The listing builds one solid part. Answer for the finished solid, in the listing's coordinates (mm). A direction names the side the tool comes from. Give positions to 0.01 mm unless a question says otherwise; leave off trailing zeros. Write each loop counter-clockwise with the first axis right and the second up, starting at its lowest first coordinate (ties: lowest second). Pieces come first, ordered by that corner, then holes. Notation, with made-up numbers: (41.25, -15) - (56.25, -15) arc R32 cw to (56.25, 14) - close; hole circle Ø10 at (24.25, 3.5). An arc over 180 degrees is marked (long way). Write each question's results on one line, items separated by ' | '. Start each with the question number.
Q1. Flat-ended cylindrical pins translate along their axes: pin 1 Ø2 at (x, z) = (-1.5, 4.5) entering from -Y; pin 2 Ø1.5 at (x, z) = (28, 3) entering from +Y. Find the tip coordinate at first contact, or state that the pin passes through.
Q2. Section C-C (z = 1.9) is taken. Determine the outline of the cut face in (x, y).
Q3. Find the intervals of material crossed by probe 1 along Y at (x, z) = (0, 2.65); probe 2 along X at (y, z) = (0.5, 0.45); probe 3 along Y at (x, z) = (-2.5, 2.2), in increasing order.
Q4. Section A-A (x = 0) is taken. Determine the outline of the cut face in (y, z).
Q5. Section B-B (y = 2) is taken. Determine the outline of the cut face in (x, z).
Q6. For a pull along Y with two mould halves and no side action, classify faces 4 (the face through (23.142, -22, 2)), 5 (the face through (27, 28.492, 2)), 6 (the face through (9.67, -18.593, 2.535)) as pulls with the +Y half, pulls with the -Y half, needs draft (parallel to the pull), parting line crosses it, or undercut.
Q7. For faces 1 (the face through (23.142, 23, 2)), 2 (the face through (27, -27.794, 2)), 3 (the face through (-19.24, 19.96, 2.54)), determine the directions among +Z, -Z, +X, -X, +Y, -Y from which every point of the face is accessible in a straight line to the end or side of a thin tool.
```python
from build123d import *

# Parameters (mm, degrees)
F0_R     = 28.827608
F1_DEPTH = 5
F2_R     = 20.957085
F3_DEPTH = 5
F4_W     = 7.907964
F4_H     = 56.286104
F5_DEPTH = 5
F6_R     = 2.590527
F7_DEPTH = 5


with BuildPart() as f1:
    # F0 (on Top) → F1 (new body)
    with BuildSketch(Plane.XY):
        with Locations((0, 0.851326)):
            Circle(F0_R)
    extrude(amount=F1_DEPTH)

    # F2 (on face) → F3 (cut)
    with BuildSketch(Plane.XY.offset(5)):
        Circle(F2_R)
    extrude(amount=-F3_DEPTH, mode=Mode.SUBTRACT)

    # F4 (on Top) → F5 (join)
    with BuildSketch(Plane.XY):
        with Locations((27.096411, 0.348881)):
            Rectangle(F4_W, F4_H)
    extrude(amount=F5_DEPTH)

    # F6 (on face) → F7 (cut)
    with BuildSketch(Plane.XY.offset(5)):
        with Locations((-16.652713, 19.845931)):
            Circle(F6_R)
    extrude(amount=-F7_DEPTH, mode=Mode.SUBTRACT)


solid = f1.part
```
Answers below:
1) pin 1: stops at y = -27.97 | pin 2: stops at y = 28.49
2) outline: (23.14, -27.79) - (31.05, -27.79) - (31.05, 28.49) - (23.14, 28.49) - (23.14, 18.04) arc R28.83 ccw (long way) to (23.14, -16.34) - close; hole circle Ø41.91 at (0, 0); hole circle Ø5.18 at (-16.65, 19.85)
3) probe 1: y = -27.98 to -20.96, 20.96 to 29.68 | probe 2: x = -28.83 to -20.95, 20.95 to 31.05 | probe 3: y = -27.87 to -20.81, 20.81 to 29.57
4) outline: (-27.98, 0) - (-20.96, 0) - (-20.96, 5) - (-27.98, 5) - close; (20.96, 0) - (29.68, 0) - (29.68, 5) - (20.96, 5) - close
5) outline: (-28.8, 0) - (-20.86, 0) - (-20.86, 5) - (-28.8, 5) - close; (20.86, 0) - (31.05, 0) - (31.05, 5) - (20.86, 5) - close
6) face 4: needs draft | face 5: pulls with the +Y half | face 6: undercut
7) face 1: +Z, -Z, +Y | face 2: +Z, -Z, +X, -Y | face 3: +Z, -Z
